Can you work these out from the drawing? Everything is in mm from the part's minimum corner. Round coordinates to 2 decimals unless told otherwise and drop trailing zeros. Write each loop counter-clockwise with the first axis right and the second up, starting at its lowest first coordinate (ties: lowest second). Pieces come first, ordered by that corner, then holes. Notation, with made-up numbers: (-11, 70.25) - (39, 70.25) arc R21 ccw to (39, 88.25) - close; hole circle Ø10 at (33.5, -32). An arc over 180 degrees is marked (long way). One line per item, written item: value. Start each with the question number.
(1) Thinking about a two-plate mould opening in X: for the marked faces 1, 2, 3 and 4, which applies, +X half, -X half, draft (parallel to the pull), parting line (faces both ways), or undercut?
(2) I want a section at D-D on z = 17. List the corners of the cut face in (x, y) for me, plus the area to 3 significant figures.
(3) If I drill on L1, parallel to Y at x = 4, z = 5.25; L2, parallel to Y at x = 4.75, z = 6; L3, parallel to X at y = 2.5, z = 24.5, over which ranges is the centre line in solid material (lowest first)? Write a range as from..to.
(4) I'm going to push flat-ended pins straight in: pin 1 Ø3 at (x, y) = (4, 4) entering from -Z; pin 2 Ø2.5 at (x, y) = (4, 4) entering from +Z. Where does each tip first touch, or does it pass through?
(5) I want a section at C-C on z = 6.5. List the corners of the cut face in (x, y) for me, plus the area to 3 significant figures.
(6) I want a section at A-A on y = 4. List the corners of the cut face in (x, z) for me, plus the area to 3 significant figures.
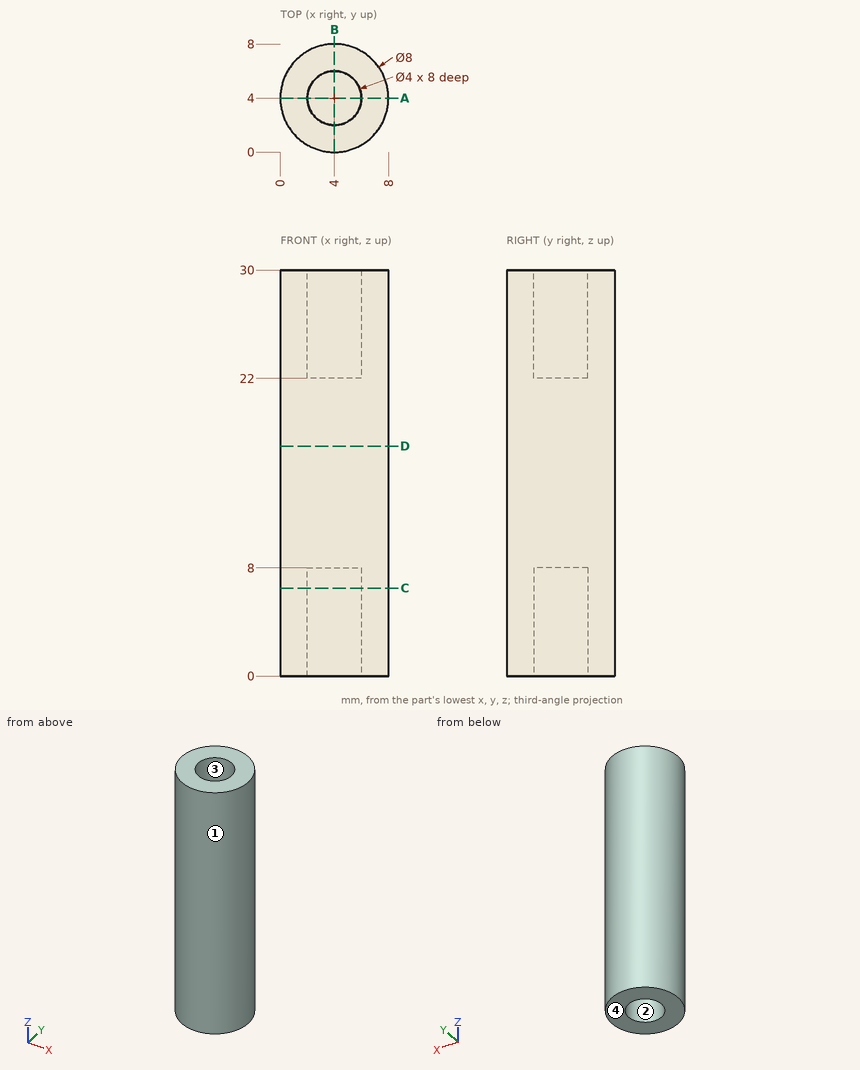
Established:
1. face 1: parting line
1. face 2: undercut
1. face 3: undercut
1. face 4: draft
2. outline: circle Ø8 at (4, 4)
2. area: 50.3 mm2
3. L1: 0..2, 6..8
3. L2: 0.07..2.15, 5.85..7.93
3. L3: 0.29..2.68, 5.32..7.71
4. pin 1: z = 8
4. pin 2: z = 22
5. outline: circle Ø8 at (4, 4); hole circle Ø4 at (4, 4)
5. area: 37.7 mm2
6. outline: (0, 0) - (2, 0) - (2, 8) - (6, 8) - (6, 0) - (8, 0) - (8, 30) - (6, 30) - (6, 22) - (2, 22) - (2, 30) - (0, 30) - close
6. area: 176 mm2
